Read the model definition and answer for the solid it produces. Units are mm, in the model's axes. Coordinates: 2 decimals unless noted, no trailing zeros. Order: outer loops, then holes, each group sorted by start corner. A loop starts at its lowest first (then second) coordinate and runs counter-clockwise, first axis right, second up. Notation, with made-up numbers: M 31.5,42 L 87.5,42 A29 ccw 87.5,64 Z; hole C -14,74.5 d6. An arc over 180 degrees is marked long. One line per question, with ' | ' between items. Start each with the question number.
1) Find section A-A, the plane x = 0.4. Write down the section's boundary in (y, z).
2) Consider probe 1 along Y at (x, z) = (0.35, -76.5); probe 2 along Z at (x, y) = (0.5, -231); probe 3 along Y at (x, z) = (1.45, -228.5). Determine where each line is inside the solid, lowest interval first.
3) Find section B-B, the plane z = -150. Write down the section's boundary in (x, y).
4) Given P1, Ø0.8, axis at x = 0.5, y = -287.5, coming from the +Z side, flat-ended and moving along its own axis, determine where the tip first touches the part or whether it passes through.
5) Find section C-C, the plane y = -240. Write down the section's boundary in (x, z), plus the area to 3 significant figures.
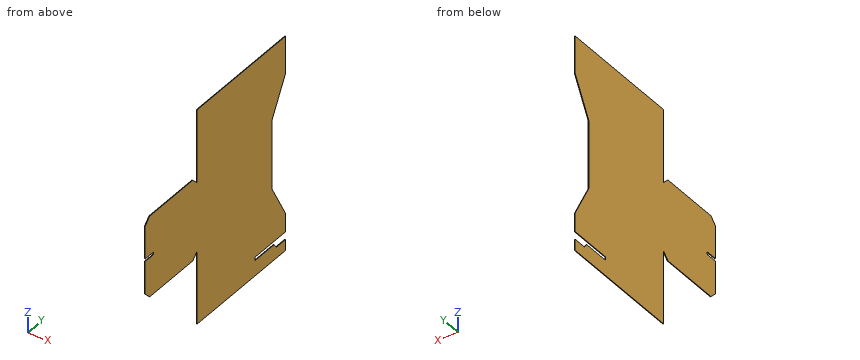
from build123d import *

# Parameters (mm, degrees)
F0_W     = 246.5
F0_H     = 160
F1_DEPTH = 1.5


with BuildPart() as f1:
    # F0 (on Right) → F1 (new body)
    with BuildSketch(Plane.YZ):
        with BuildLine():
            Line((-295.25, -80), (-123.25, -80))
            Line((-123.25, -80), (-123.25, 80))
            Line((-123.25, 80), (-123.695542, 80))
            Line((-123.695542, 80), (-295.25, 80))
            Line((-295.25, 80), (-295.25, 3))
            Line((-295.25, 3), (-270.25, 3))
            ThreePointArc((-270.25, 3), (-267.25, 0), (-270.25, -3))
            Line((-270.25, -3), (-295.25, -3))
            Line((-295.25, -3), (-295.25, -80))
        make_face()
        Polygon((-123.695542, 80), (-123.25, 80), (-138.25, 95), (-280.25, 95), (-295.25, 80), align=None)
        Polygon((-138.25, -95), (-123.25, -80), (-295.25, -80), (-280.25, -95), align=None)
        Rectangle(F0_W, F0_H)
        Polygon((-123.25, 80), (123.25, 80), (168.25, 164), (168.25, 252), (-123.25, 252), align=None)
        Polygon((168.25, -164), (123.25, -80), (-123.25, -80), (-123.25, -252), (168.25, -252), (168.25, -226), (138.25, -226), (130.25, -216), (68.25, -216), (68.25, -208), (168.25, -208), align=None)
    extrude(amount=F1_DEPTH)


solid = f1.part
Report:
1) outline: M -295.25,-80 L -280.25,-95 L -138.25,-95 L -123.25,-80 L -123.25,-252 L 168.25,-252 L 168.25,-226 L 138.25,-226 L 130.25,-216 L 68.25,-216 L 68.25,-208 L 168.25,-208 L 168.25,-164 L 123.25,-80 L 123.25,80 L 168.25,164 L 168.25,252 L -123.25,252 L -123.25,80 L -138.25,95 L -280.25,95 L -295.25,80 L -295.25,3 L -270.25,3 A3 cw -270.25,-3 L -295.25,-3 Z
2) probe 1: y = -295.25 to 123.25 | probe 2: z = -95 to 95 | probe 3: y = -123.25 to 168.25
3) outline: M 0,-123.25 L 1.5,-123.25 L 1.5,160.75 L 0,160.75 Z
4) P1: stops at z = 88.15
5) outline: M 0,-95 L 1.5,-95 L 1.5,95 L 0,95 Z | area: 285 mm^2
